```python
from build123d import *

# Parameters (mm, degrees)
BOSS_EXTRUDE1_DEPTH = 5
CUT_EXTRUDE1_REACH  = 18.882
SKETCH2_R           = 1.4
FILLET1_R           = 2
FILLET2_R           = 2


with BuildPart() as part:
    # Sketch1 → Boss-Extrude1 (new, symmetric)
    with BuildSketch(Plane.XY):
        Polygon((-14, 0), (-6.963555158, 0), (-4.779733752, 6), (4.779733752, 6), (6.963555158, 0), (14, 0), (14, 3), (8, 3), (6.180148829, 8), (-6.180148829, 8), (-8, 3), (-14, 3), align=None)
    extrude(amount=BOSS_EXTRUDE1_DEPTH, both=True)

    # Sketch2 → Cut-Extrude1 (cut, up to next)
    with BuildSketch(Plane.XZ, mode=Mode.PRIVATE) as cut_extrude1_sk1:
        with Locations(Location((-11, 0, 0), (0, 0, 270))):
            Circle(SKETCH2_R)
    cut_extrude1_tool1 = extrude(cut_extrude1_sk1.sketch, amount=-CUT_EXTRUDE1_REACH, mode=Mode.PRIVATE) & part.part
    # Sketch2 → Cut-Extrude1 (cut, up to next)
    with BuildSketch(Plane.XZ, mode=Mode.PRIVATE) as cut_extrude1_sk2:
        with Locations(Location((11, 0, 0), (0, 0, 270))):
            Circle(SKETCH2_R)
    cut_extrude1_tool2 = extrude(cut_extrude1_sk2.sketch, amount=-CUT_EXTRUDE1_REACH, mode=Mode.PRIVATE) & part.part
    add(cut_extrude1_tool1.solids().sort_by_distance((-11, 0, 0))[0], mode=Mode.SUBTRACT)
    add(cut_extrude1_tool2.solids().sort_by_distance((11, 0, 0))[0], mode=Mode.SUBTRACT)

    # Fillet1
    fillet1_edges = [part.edges().sort_by_distance(p)[0] for p in [
        (-5.871644455, 3, 5),
        (5.871644455, 3, -5),
        (0, 6, -5),
        (-5.871644455, 3, -5),
        (0, 6, 5),
        (5.871644455, 3, 5),
    ]]
    fillet(fillet1_edges, radius=FILLET1_R - 0.0001)  # a hair under: the kernel refuses the full size

    # Fillet2
    fillet2_edges = [part.edges().sort_by_distance(p)[0] for p in [
        (14, 1.5, -5),
        (-14, 1.5, -5),
        (14, 1.5, 5),
        (-14, 1.5, 5),
    ]]
    fillet(fillet2_edges, radius=FILLET2_R)


solid = part.part
```
Could you check a few things on this model? Use its own coordinates, in mm. A direction names the side the tool comes from. Coordinates: 2 decimals unless noted, no trailing zeros. Order: outer loops, then holes, each group sorted by start corner. A loop starts at its lowest first (then second) coordinate and runs counter-clockwise, first axis right, second up. Notation, with made-up numbers: M 84,62 L 120,62 A18 cw 120,68 Z; hole C 60.25,38 d2. An arc over 180 degrees is marked long. Use one line per item in the form item = value. Start each with the question number.
1. We'd pull the mould along X, two halves only. Please class faces 4 (the flat face through (-9, 2, -5)), 5 (the cylindrical face through (-13.4, 1.48, -4.43)), 6 (the cylindrical face through (13.4, 1.52, 4.43)), 7 (the cylindrical face through (0.09, 6.6, -4.43)): +X half, -X half, draft (parallel to the pull), parting line (faces both ways), or undercut.
2. Please list where these lines run through material, in increasing order: line 1 (X direction, y = 2.15, z = 0); line 2 (X direction, y = 1.9, z = 0); line 3 (Y direction, x = -10.5, z = -1.75).
3. For pin 1 (1.8 mm diameter, centred on x = 11.5, z = -2.5, fed in from +Y), with a flat end and sliding along its axis, tell me the tip position at first contact or that it passes through.
4. Suppose I cut it at D-D on y = 1. Count the separate pieces of the cut face and the enclosed holes in it, then the cut area to 3 significant figures.
5. Suppose I cut it at B-B on x = 11. Write out the boundary of the cut face in (y, z), then the cut area to 3 significant figures.
6. On a 3-axis mill with a long thin cutter (end or side, diameter ignored), from which of +Z, -Z, +X, -X, +Y, -Y can I reach the whole of each face in a straight line? I mean faces 1 (the cylindrical face through (0.09, 6.6, 4.43)), 2 (the flat face through (-5.887, 2.958, 0.042)), 3 (the flat face through (-7.08, 5.53, 0.07)). Say none if no direction works.
7. Suppose I cut it at A-A on z = 0. Write out the boundary of the cut face in (x, y).
Geometry says:
q1.face_4 = draft
q1.face_5 = -X half
q1.face_6 = +X half
q1.face_7 = undercut
q2.line_1 = -14 to -12.4, -9.6 to -6.18, 6.18 to 9.6, 12.4 to 14
q2.line_2 = -14 to -12.4, -9.6 to -6.27, 6.27 to 9.6, 12.4 to 14
q2.line_3 = 0 to 3
q3.pin_1 = 3
q4.separate_pieces = 2
q4.enclosed_holes = 2
q4.area = 129 mm^2
q5.outline = M 0,-5 L 3,-5 L 3,-1.4 L 0,-1.4 Z; M 0,1.4 L 3,1.4 L 3,5 L 0,5 Z
q5.area = 21.6 mm^2
q6.face_1 = +Z, -Y
q6.face_2 = +Z, -Z, -Y
q6.face_3 = +Z, -Z, -X, +Y
q7.outline = M -14,0 L -12.4,0 L -12.4,3 L -14,3 Z; M -9.6,0 L -6.96,0 L -4.78,6 L 4.78,6 L 6.96,0 L 9.6,0 L 9.6,3 L 8,3 L 6.18,8 L -6.18,8 L -8,3 L -9.6,3 Z; M 12.4,0 L 14,0 L 14,3 L 12.4,3 Z
